```python
from build123d import *

# Parameters (mm, degrees)
F0_W     = 85.7
F0_H     = 85.7
F0_W_2   = 75.7
F0_H_2   = 75.7
F1_DEPTH = 50
F2_DEPTH = 5
F4_DEPTH = 20
F5_R     = 2.54


with BuildPart() as f1:
    # F0 (on Top) → F1 (new body)
    with BuildSketch(Plane.XY):
        Rectangle(F0_W, F0_H)
        Rectangle(F0_W_2, F0_H_2, mode=Mode.SUBTRACT)
    extrude(amount=F1_DEPTH)

    # F0 (on Top) → F2 (join)
    with BuildSketch(Plane.XY):
        Rectangle(F0_W_2, F0_H_2)
    extrude(amount=F2_DEPTH)

    # F3 (on face) → F4 (cut)
    with BuildSketch(Plane.XZ.offset(42.85)):
        with BuildLine():
            ThreePointArc((-8.123884, 15), (0, 6.876116), (8.123884, 15))
            Line((8.123884, 15), (-8.123884, 15))
        make_face()
        with BuildLine():
            Line((-8.123884, 15), (8.123884, 15))
            ThreePointArc((8.123884, 15), (0, 23.123884), (-8.123884, 15))
        make_face()
        with BuildLine():
            Line((8.123884, 15), (8.123884, 50))
            Line((8.123884, 50), (-8.123884, 50))
            Line((-8.123884, 50), (-8.123884, 15))
            ThreePointArc((-8.123884, 15), (0, 23.123884), (8.123884, 15))
        make_face()
    extrude(amount=-F4_DEPTH, mode=Mode.SUBTRACT)

    # F5
    f5_edges = [f1.edges().sort_by_distance(p)[0] for p in [
        (0, -42.85, 6.876116),
        (8.123884, -42.85, 32.5),
        (25.486942, -42.85, 50),
        (-25.486942, -42.85, 50),
        (42.85, 0, 50),
        (0, 42.85, 50),
        (-42.85, 0, 50),
        (-8.123884, -42.85, 32.5),
    ]]
    fillet(f5_edges, radius=F5_R)


solid = f1.part
```
Here's how the part is built. I have some questions about the finished solid (model axes, mm). A direction names the side the tool comes from. Round coordinates to 2 decimals unless told otherwise and drop trailing zeros. Write each loop counter-clockwise with the first axis right and the second up, starting at its lowest first coordinate (ties: lowest second). Pieces come first, ordered by that corner, then holes.
Q1. Please list where this line runs through material, in increasing order: probe 1 along X at (y, z) = (-26, 39).
Q2. If we section it at B-B on x = 0: Write out the boundary of the cut face in (y, z), plus the area to 3 significant figures.
Q3. Will this pin go through, and if not, where does the flat tip stop? P1, Ø10, axis at x = -8.5, y = -20, coming from the +Z side.
Q4. If we section it at C-C on z = 37: Write out the boundary of the cut face in (x, y).
Q5. If we mould it in two halves opening along Y, with no side actions, what happens to faces 1 (the cylindrical face through (8.89, -42.13, 32.75)), 2 (the flat face through (37.85, -1, 27)), 3 (the flat face through (42.85, -1, 23)), 4 (the cylindrical face through (0.6, 42.126, 49.236))? For each: +Y half, -Y half, draft (parallel to the pull), parting line (faces both ways), or undercut.
Q6. If we section it at A-A on y = -20: Write out the boundary of the cut face in (x, z), plus the area to 3 significant figures.
Q7. Which directions (+Z, -Z, +X, -X, +Y, -Y) give clear straight access to the entire face, cutting with the end or side of a thin tool? Please do faces 5 (the flat face through (-1, 1, 5)), 6 (the cylindrical face through (42.126, 0.6, 49.236)), 7 (the cylindrical face through (-8.89, -42.13, 32.25)).
Answer below:
1. probe 1: x = -42.85 to -37.85, 37.85 to 42.85
2. outline: (-42.85, 0) - (42.85, 0) - (42.85, 47.46) arc R2.54 ccw to (40.31, 50) - (37.85, 50) - (37.85, 5) - (-37.85, 5) - (-37.85, 6.88) - (-40.31, 6.88) arc R2.54 ccw to (-42.85, 4.34) - close
2. area: 660 mm2
3. P1: stops at z = 5
4. outline: (-42.85, -42.85) - (-10.66, -42.85) arc R2.54 ccw to (-8.12, -40.31) - (-8.12, -37.85) - (-37.85, -37.85) - (-37.85, 37.85) - (37.85, 37.85) - (37.85, -37.85) - (8.12, -37.85) - (8.12, -40.31) arc R2.54 ccw to (10.66, -42.85) - (42.85, -42.85) - (42.85, 42.85) - (-42.85, 42.85) - close
5. face 1: -Y half
5. face 2: undercut
5. face 3: draft
5. face 4: +Y half
6. outline: (-42.85, 0) - (42.85, 0) - (42.85, 47.46) arc R2.54 ccw to (40.31, 50) - (37.85, 50) - (37.85, 5) - (-37.85, 5) - (-37.85, 50) - (-40.31, 50) arc R2.54 ccw to (-42.85, 47.46) - close
6. area: 876 mm2
7. face 5: +Z
7. face 6: +Z, +X, +Y, -Y
7. face 7: +Z, -Y
